from build123d import *

# Parameters (mm, degrees)
CYLINDER1984_R               = 1.5
CYLINDER1984_DEPTH           = 50
COMPOUND1069_PLACEMENT_ANGLE = 225
CYLINDER1985_R               = 1.5
CYLINDER1985_DEPTH           = 50
COMPOUND1070_PLACEMENT_ANGLE = 225
CYLINDER1983_R               = 74
CYLINDER1983_DEPTH           = 40
BOX984_W                     = 42
BOX984_H                     = 8
BOX984_DEPTH                 = 10
COMPOUND1068_PLACEMENT_ANGLE = 225


with BuildPart() as compound1069:
    # Cylinder1984 → Cylinder1984 (new body)
    with BuildSketch(Plane(origin=(9, 100, 59), x_dir=(1, 0, 0), z_dir=(0, -1, 0))):
        Circle(CYLINDER1984_R)
    extrude(amount=CYLINDER1984_DEPTH)


with BuildPart() as compound1069_1:
    # Compound1069 placement: moved
    add(compound1069.part.rotate(Axis((0, 0, 0), (0, 0, 1)), COMPOUND1069_PLACEMENT_ANGLE))


with BuildPart() as compound1071:
    # Cylinder1985 → Cylinder1985 (new body)
    with BuildSketch(Plane(origin=(-9, 100, 59), x_dir=(1, 0, 0), z_dir=(0, -1, 0))):
        Circle(CYLINDER1985_R)
    extrude(amount=CYLINDER1985_DEPTH)


with BuildPart() as compound1071_1:
    # Compound1070 placement: moved
    add(compound1071.part.rotate(Axis((0, 0, 0), (0, 0, 1)), COMPOUND1070_PLACEMENT_ANGLE))

    # Compound1071: union Compound1069
    add(compound1069_1.part)


with BuildPart() as compound1071_2:
    # Compound1071 placement: moved
    add(compound1071_1.part.moved(Location((0, 0, 1))))


with BuildPart() as obj1:
    # Cylinder1983 → Cylinder1983 (new body)
    with BuildSketch(Plane.XY.offset(44)):
        Circle(CYLINDER1983_R)
    extrude(amount=CYLINDER1983_DEPTH)


with BuildPart() as cut668:
    # Box984 → Box984 (new body)
    with BuildSketch(Plane(origin=(-21, -23, 22), x_dir=(1, 0, 0), z_dir=(0, 0, 1))):
        with Locations((21, 4)):
            Rectangle(BOX984_W, BOX984_H)
    extrude(amount=BOX984_DEPTH)


with BuildPart() as cut668_1:
    # Compound1068 placement: moved
    add(cut668.part.moved(Location((63.64, -63.64, 43))).rotate(Axis((63.64, -63.64, 43), (0, 0, 1)), COMPOUND1068_PLACEMENT_ANGLE))

    # Cut667: cut obj1
    add(obj1.part, mode=Mode.SUBTRACT)


with BuildPart() as cut668_2:
    # Cut667 placement: moved
    add(cut668_1.part.moved(Location((0, 0, -10))))

    # Cut668: cut Compound1071
    add(compound1071_2.part, mode=Mode.SUBTRACT)


solid = cut668_2.part
Design review of the part built by this model. Coordinates are the model's own, in mm. Round coordinates to 2 decimals unless told otherwise and drop trailing zeros. Write each loop counter-clockwise with the first axis right and the second up, starting at its lowest first coordinate (ties: lowest second). Pieces come first, ordered by that corner, then holes. Notation, with made-up numbers: (30, -31) - (39, -31) arc R17 ccw to (39, -20) - close; hole circle Ø1 at (55, 44). An arc over 180 degrees is marked (long way). Return JSON: item names as keys, results as strings. Group by question number.
Item 1: The part is to be moulded in two halves that separate along Z. For faces 1 (the face through (45.05, -59.8, 60.45)), 2 (the face through (53, -52, 55)), 3 (the face through (36.7, -66.4, 59.9)), 4 (the face through (59.846, -44.999, 60.066)), say which applies: pulls with the +Z half, pulls with the -Z half, needs draft (parallel to the pull), parting line crosses it, or undercut.
Item 2: Insertion check: P1, Ø2, axis at x = 50.5, z = 61, coming from the -Y side; P2, Ø4, axis at y = -57, z = 57.5, coming from the +X side; P3, Ø2, axis at y = -44, z = 58.5, coming from the +X side. Each pin has a flat end and moves straight along its axis. Give the tip position at first contact, or say it passes through.
Item 3: We need section B-B on y = -42. Write out the cut boundary in (x, z), and give its area (3 significant figures).
Item 4: For probe 1 along X at (y, z) = (-63.5, 57.5); probe 2 along X at (y, z) = (-55, 64.5); probe 3 along Y at (x, z) = (38.5, 62), list the stretches that pass through material, from the lowest coordinate up. Write a range as [from, to].
Item 5: We need section A-A on z = 61. Write out the cut boundary in (x, y).
Item 6: We need section C-C on z = 57.75. Write out the cut boundary in (x, y).
Model answer:
{
 "1": {"face 1": "undercut", "face 2": "pulls with the -Z half", "face 3": "needs draft", "face 4": "undercut"},
 "2": {"P1": "stops at y = -56.57", "P2": "stops at x = 51.07", "P3": "stops at x = 63.07"},
 "3": {"outline": "(60.93, 55) - (64.07, 55) - (64.07, 65) - (60.93, 65) - close", "area": "31.4 mm²"},
 "4": {"probe 1": "x = [38, 42.57]", "probe 2": "x = [49.51, 51.07]", "probe 3": "y = [-67.57, -63.2]"},
 "5": {"outline": "(35.33, -65.02) - (38.18, -67.88) - (45.88, -60.19) - (44.68, -58.99) arc R74 cw to start; (46.45, -57.6) - (47.46, -58.61) - (58.61, -47.46) - (57.6, -46.45) arc R74 cw to start; (58.99, -44.68) - (60.19, -45.88) - (67.88, -38.18) - (65.02, -35.33) arc R74 cw to start"},
 "6": {"outline": "(35.33, -65.02) - (38.18, -67.88) - (67.88, -38.18) - (65.02, -35.33) arc R74 cw to start"}
}
